Input: part model. Units: mm. Frame: model coordinates. A direction names the side the tool comes from. Round coordinates to 2 decimals unless told otherwise and drop trailing zeros. Write each loop counter-clockwise with the first axis right and the second up, starting at its lowest first coordinate (ties: lowest second). Pieces come first, ordered by that corner, then holes. Notation, with made-up numbers: M 71,76 L 88,76 A8 cw 88,87 Z; hole C 25,30.25 d7. An arc over 180 degrees is marked long. Write each question's results on one line, items separated by ' | '. Start each with the question number.
```python
from build123d import *

# Parameters (mm, degrees)
SKETCH_1_W               = 40
SKETCH_1_H               = 40
EXTRUDE_1_DEPTH          = 7
SKETCH_2_R               = 18
EXTRUDE_2_DEPTH          = 26
SKETCH_3_R               = 20
EXTRUDE_3_DEPTH          = 54.5
SKETCH_4_W               = 2.306133039
SKETCH_4_H               = 0.5
SKETCH_5_R               = 13
EXTRUDE_4_DEPTH          = 2
SKETCH_6_R               = 6
EXTRUDE_5_DEPTH          = 1
SKETCH_7_R               = 5
EXTRUDE_6_DEPTH          = 23
CHAMFER_1_SIZE           = 2
CHAMFER_2_SIZE           = 0.5
SKETCH_8_R               = 1.75
CUT_EXTRUDE_1_DEPTH      = 20
PATTERN_CIRCULAR_1_COUNT = 4
SKETCH_9_R               = 11
CUT_EXTRUDE_2_DEPTH      = 3
SKETCH_10_R              = 2.5
CUT_EXTRUDE_3_DEPTH      = 23
PATTERN_CIRCULAR_2_COUNT = 4
CUT_EXTRUDE_4_DEPTH      = 2.5


with BuildPart() as part:
    # 草图1 → 凸台-拉伸1 (new body)
    with BuildSketch(Plane.XY):
        Rectangle(SKETCH_1_W, SKETCH_1_H)
    extrude(amount=EXTRUDE_1_DEPTH)

    # 草图2 → 凸台-拉伸2 (add)
    with BuildSketch(Plane.XY.offset(7)):
        Circle(SKETCH_2_R)
    extrude(amount=-EXTRUDE_2_DEPTH)

    # 草图3 → 凸台-拉伸3 (add)
    with BuildSketch(Plane(origin=(0, 0, -19), x_dir=(-1, 0, 0), z_dir=(0, 0, -1))):
        Circle(SKETCH_3_R)
    extrude(amount=EXTRUDE_3_DEPTH)

    # 草图4 → 切除-旋转1 (revolve, cut)
    with BuildSketch(Plane(origin=(0, 0, 0), x_dir=(1, 0, 0), z_dir=(0, 1, 0))):
        with Locations((20.65306652, 21.25)):
            Rectangle(SKETCH_4_W, SKETCH_4_H)
    revolve(axis=Axis((0, 0, 0), (0, 0, -1)), mode=Mode.SUBTRACT)

    # 草图5 → 凸台-拉伸4 (add)
    with BuildSketch(Plane(origin=(0, 0, -73.5), x_dir=(-1, 0, 0), z_dir=(0, 0, -1))):
        Circle(SKETCH_5_R)
    extrude(amount=EXTRUDE_4_DEPTH)

    # 草图6 → 凸台-拉伸5 (add)
    with BuildSketch(Plane(origin=(0, 0, -75.5), x_dir=(-1, 0, 0), z_dir=(0, 0, -1))):
        Circle(SKETCH_6_R)
    extrude(amount=EXTRUDE_5_DEPTH)

    # 草图7 → 凸台-拉伸6 (add)
    with BuildSketch(Plane(origin=(0, 0, -76.5), x_dir=(-1, 0, 0), z_dir=(0, 0, -1))):
        Circle(SKETCH_7_R)
    extrude(amount=EXTRUDE_6_DEPTH)

    # 倒角1
    chamfer_1_edges = [part.edges().sort_by_distance(p)[0] for p in [
        (20, -20, 3.5),
        (-20, -20, 3.5),
        (-20, 20, 3.5),
        (20, 20, 3.5),
    ]]
    chamfer(chamfer_1_edges, length=CHAMFER_1_SIZE)

    # 倒角2
    chamfer_2_edges = [part.edges().sort_by_distance(p)[0] for p in [
        (20, 0, -19),
        (20, 0, -73.5),
        (6, 0, -76.5),
        (5, 0, -99.5),
    ]]
    chamfer(chamfer_2_edges, length=CHAMFER_2_SIZE)

    # 草图8 → 切除-拉伸1 (cut)
    with BuildSketch(Plane.XY.offset(7)):
        with Locations((-15.5, 15.5)):
            Circle(SKETCH_8_R)
    cut_extrude_1 = extrude(amount=-CUT_EXTRUDE_1_DEPTH, mode=Mode.SUBTRACT)

    # 阵列(圆周)1: 切除-拉伸1 ×4 about axis
    pattern_circular_1_axis = Axis((0, 0, 0), (0, 0, 1))
    for i in range(1, PATTERN_CIRCULAR_1_COUNT):
        add(cut_extrude_1.rotate(pattern_circular_1_axis, i * 360 / PATTERN_CIRCULAR_1_COUNT), mode=Mode.SUBTRACT)

    # 草图9 → 切除-拉伸2 (cut)
    with BuildSketch(Plane.XY.offset(7)):
        Circle(SKETCH_9_R)
    extrude(amount=-CUT_EXTRUDE_2_DEPTH, mode=Mode.SUBTRACT)

    # 草图10 → 切除-拉伸3 (cut)
    with BuildSketch(Plane.XY.offset(4)):
        Circle(SKETCH_10_R)
    extrude(amount=-CUT_EXTRUDE_3_DEPTH, mode=Mode.SUBTRACT)

    # 草图11 → M4 螺纹孔1 (revolve, cut)
    with BuildSketch(Plane(origin=(-12.02081528, 12.02081528, -73.5), x_dir=(0, 1, 0), z_dir=(1, 0, 0))):
        Polygon((0, 0), (0, 10.991420021), (1.65, 10), (1.65, 0), align=None)
    hole_wizard_m4_1 = revolve(axis=Axis((-12.02081528, 12.02081528, -79.85), (0, 0, 1)), mode=Mode.SUBTRACT)

    # 阵列(圆周)2: M4 螺纹孔1 ×4 about axis
    pattern_circular_2_axis = Axis((0, 0, 0), (0, 0, 1))
    for i in range(1, PATTERN_CIRCULAR_2_COUNT):
        add(hole_wizard_m4_1.rotate(pattern_circular_2_axis, i * 360 / PATTERN_CIRCULAR_2_COUNT), mode=Mode.SUBTRACT)

    # 草图13 → 切除-拉伸4 (cut)
    with BuildSketch(Plane(origin=(0, 5, 0), x_dir=(1, 0, 0), z_dir=(0, 1, 0))):
        with BuildLine():
            Line((1.5, 94.5), (1.5, 81.5))
            ThreePointArc((1.5, 81.5), (0, 80), (-1.5, 81.5))
            Line((-1.5, 81.5), (-1.5, 94.5))
            ThreePointArc((-1.5, 94.5), (0, 96), (1.5, 94.5))
        make_face()
    extrude(amount=-CUT_EXTRUDE_4_DEPTH, mode=Mode.SUBTRACT)


solid = part.part
```
1. Contact query for flat-ended pins moving along their axis: P1, Ø5.5, axis at x = 15.5, y = 15.5, coming from the -Z side; P2, Ø3, axis at x = 15.5, y = -15.5, coming from the -Z side; P3, Ø8, axis at y = 5, z = -18, coming from the +X side; P4, Ø17.5, axis at x = 1, y = 1, coming from the +Z side. Output: stop coordinate, or through.
2. Draft query along Z for faces 1 (the face through (0, 4, -96)), 2 (the face through (0, 4, -80)), 3 (the face through (0, 20, 3)), 4 (the face through (-11.7, -12, -62.7)). Return one class per face: +Z half, -Z half, draft (parallel to the pull), parting line (faces both ways), or undercut.
3. Cut plane A-A on z = -8. Output: boundary loops of the cut face in (x, y).
4. Line query: L1, parallel to X at y = -15.5, z = 5; L2, parallel to Y at x = 0, z = -12.25; L3, parallel to Y at x = 0, z = 5. Output: solid intervals per line, ascending. Write a range as from..to.
5. Access query for faces 5 (the face through (-2.38, -10.74, 5.52)), 6 (the face through (10.71, 11.02, -68.57)), 7 (the face through (19, 19, 3)), 8 (the face through (0, -20, 3)), 9 (the face through (-5, 18, 0)). Directions: +Z, -Z, +X, -X, +Y, -Y. A direction counts if a zero-diameter tool reaches every point of the face in a straight line with its end or side. Return the directions, or none.
6. Cut plane C-C on y = -15.5. Give the number of separate pieces and of enclosed holes in the cut face, and give its area (3 significant figures).
7. Cut plane B-B on z = -52.5. Output: boundary loops of the cut face in (x, y), and give its area (3 significant figures).
Answers follow:
1) P1: stops at z = -73.5 | P2: passes through | P3: stops at x = 19.96 | P4: stops at z = 4
2) face 1: undercut | face 2: undercut | face 3: draft | face 4: -Z half
3) outline: C 0,0 d36; hole C 0,0 d5
4) L1: x = -20..-17.25, -13.75..13.75, 17.25..20 | L2: y = -18..-2.5, 2.5..18 | L3: y = -20..-11, 11..20
5) face 5: +Z | face 6: -Z | face 7: +Z, -Z, +X, +Y | face 8: +Z, -Z, +X, -X, -Y | face 9: none
6) separate pieces: 3 | enclosed holes: 0 | area: 1,950 mm2
7) outline: C 0,0 d40 | area: 1,260 mm2
